```python
from build123d import *

# Parameters (mm, degrees)
ESBO_O1_W                  = 100
ESBO_O1_H                  = 100
RESSALTO_EXTRUS_O1_DEPTH   = 1.5
ESBO_O2_R                  = 1.5
ESBO_O2_W                  = 40
ESBO_O2_H                  = 3
CORTE_EXTRUS_O1_DEPTH      = 71.774289117
ESBO_O3_W                  = 3
ESBO_O3_H                  = 34.5
RESSALTO_EXTRUS_O2_DEPTH   = 3
CUT_EXTRUDE4_DEPTH         = 73.878323252
CUT_EXTRUDE4_DEPTH_BACK    = 73.878323252
FILLET1_R                  = 5
CUT_EXTRUDE5_DEPTH         = 73.878323252
CUT_EXTRUDE5_DEPTH_BACK    = 73.878323252
SKETCH3_W                  = 3
SKETCH3_H                  = 15
SKETCH3_W_2                = 4
SKETCH3_H_2                = 3
SKETCH3_H_3                = 7
CORTE_GY_VL53L0_DEPTH      = 73.924618614
CORTE_GY_VL53L0_DEPTH_BACK = 73.924618614
CUT_EXTRUDE6_DEPTH         = 73.924618614
CUT_EXTRUDE6_DEPTH_BACK    = 73.924618614
SKETCH4_R                  = 1.1
SKETCH4_W                  = 22.5
SKETCH4_H                  = 12.2
CUT_EXTRUDE7_DEPTH         = 73.924618614
CUT_EXTRUDE7_DEPTH_BACK    = 73.924618614


with BuildPart() as part:
    # Esboço1 → Ressalto-extrusão1 (new, symmetric)
    with BuildSketch(Plane.XY):
        Rectangle(ESBO_O1_W, ESBO_O1_H)
    extrude(amount=RESSALTO_EXTRUS_O1_DEPTH, both=True)

    # Esboço2 → Corte-extrusão1 (cut, through all)
    with BuildSketch(Plane.XY.offset(1.5)):
        with Locations((-33, 11.5)):
            Circle(ESBO_O2_R)
        with Locations(Location((33, 11.5, 0), (0, 0, 180))):
            Circle(ESBO_O2_R)
        with Locations((0, -48.5)):
            Rectangle(ESBO_O2_W, ESBO_O2_H)
        with Locations((0, 11.5)):
            Rectangle(ESBO_O2_W, ESBO_O2_H)
    extrude(amount=-CORTE_EXTRUS_O1_DEPTH, mode=Mode.SUBTRACT)

    # Esboço3 → Ressalto-extrusão2 (add, through all)
    with BuildSketch(Plane.XY.offset(1.5)):
        with Locations((-51.5, -32.75)):
            Rectangle(ESBO_O3_W, ESBO_O3_H)
        with Locations((51.5, -32.75)):
            Rectangle(ESBO_O3_W, ESBO_O3_H)
        with Locations((-51.5, 32.75)):
            Rectangle(ESBO_O3_W, ESBO_O3_H)
        with Locations((51.5, 32.75)):
            Rectangle(ESBO_O3_W, ESBO_O3_H)
    extrude(amount=-RESSALTO_EXTRUS_O2_DEPTH)

    # Sketch2 → Cut-Extrude4 (cut, two sides: drawn at the far end of the back side and taken through both)
    with BuildSketch(Plane.XY.offset(-CUT_EXTRUDE4_DEPTH_BACK)):
        with BuildLine():
            Line((-0.5, -35), (0.5, -35))
            ThreePointArc((0.5, -35), (1.207106781, -35.292893219), (1.5, -36))
            Line((1.5, -36), (1.5, -40.73))
            Line((1.5, -40.73), (2.85, -40.73))
            Line((2.85, -40.73), (2.85, -43))
            Line((2.85, -43), (1.5, -43))
            Line((1.5, -43), (1.5, -47))
            Line((1.5, -47), (-1.5, -47))
            Line((-1.5, -47), (-1.5, -43))
            Line((-1.5, -43), (-2.85, -43))
            Line((-2.85, -43), (-2.85, -40.73))
            Line((-2.85, -40.73), (-1.5, -40.73))
            Line((-1.5, -40.73), (-1.5, -36))
            ThreePointArc((-1.5, -36), (-1.207106781, -35.292893219), (-0.5, -35))
        make_face()
    extrude(amount=CUT_EXTRUDE4_DEPTH + CUT_EXTRUDE4_DEPTH_BACK, mode=Mode.SUBTRACT)

    # Fillet1
    fillet1_edges = [part.edges().sort_by_distance(p)[0] for p in [
        (53, 50, 0),
        (-53, 50, 0),
    ]]
    fillet(fillet1_edges, radius=FILLET1_R)

    # Sketch3 → Cut-Extrude5 (cut, two sides: drawn at the far end of the back side and taken through both)
    with BuildSketch(Plane.XY.offset(-CUT_EXTRUDE5_DEPTH_BACK)):
        with Locations((9, -6.5)):
            Rectangle(SKETCH3_W, SKETCH3_H)
        with Locations((9, 28.5)):
            Rectangle(SKETCH3_W, SKETCH3_H)
        with Locations((-9, 28.5)):
            Rectangle(SKETCH3_W, SKETCH3_H)
        with Locations((-9, -6.5)):
            Rectangle(SKETCH3_W, SKETCH3_H)
        with Locations((0, -27.5)):
            Rectangle(SKETCH3_W_2, SKETCH3_H_2)
        Polygon((-15.196152423, -40), (-10, -37), (-8.5, -39.598076211), (-13.696152423, -42.598076211), align=None)
        Polygon((10, -37), (8.5, -39.598076211), (13.696152423, -42.598076211), (15.196152423, -40), align=None)
        with Locations((-48.5, -43.5)):
            Rectangle(SKETCH3_W, SKETCH3_H_3)
        with Locations((48.5, -43.5)):
            Rectangle(SKETCH3_W, SKETCH3_H_3)
    extrude(amount=CUT_EXTRUDE5_DEPTH + CUT_EXTRUDE5_DEPTH_BACK, mode=Mode.SUBTRACT)

    # Sketch1 → Corte Gy-VL53L0 (cut, two sides: drawn at the far end of the back side and taken through both)
    with BuildSketch(Plane(origin=(0, 0, -1.5), x_dir=(-1, 0, 0), z_dir=(0, 0, -1)).offset(-CORTE_GY_VL53L0_DEPTH_BACK)):
        with BuildLine():
            Line((-46.5, 42.530680232), (-46.495662433, 42.530680232))
            ThreePointArc((-46.495662433, 42.530680232), (-46.062649731, 42.780680232), (-46.062649731, 43.280680232))
            Line((-46.062649731, 43.280680232), (-46.64, 44.280680232))
            Line((-46.64, 44.280680232), (-45.07, 47))
            Line((-45.07, 47), (-41.93, 47))
            Line((-41.93, 47), (-40.36, 44.280680232))
            Line((-40.36, 44.280680232), (-40.937350269, 43.280680232))
            ThreePointArc((-40.937350269, 43.280680232), (-40.937350269, 42.780680232), (-40.504337567, 42.530680232))
            Line((-40.504337567, 42.530680232), (-39, 42.530680232))
            ThreePointArc((-39, 42.530680232), (-37.585786438, 41.944893794), (-37, 40.530680232))
            Line((-37, 40.530680232), (-37, 28.530680232))
            ThreePointArc((-37, 28.530680232), (-37.585786438, 27.11646667), (-39, 26.530680232))
            Line((-39, 26.530680232), (-40.504337567, 26.530680232))
            ThreePointArc((-40.504337567, 26.530680232), (-40.937350269, 26.280680232), (-40.937350269, 25.780680232))
            Line((-40.937350269, 25.780680232), (-40.36, 24.780680232))
            Line((-40.36, 24.780680232), (-41.93, 22.061360464))
            Line((-41.93, 22.061360464), (-45.07, 22.061360464))
            Line((-45.07, 22.061360464), (-46.64, 24.780680232))
            Line((-46.64, 24.780680232), (-46.062649731, 25.780680232))
            ThreePointArc((-46.062649731, 25.780680232), (-46.062649731, 26.280680232), (-46.495662433, 26.530680232))
            Line((-46.495662433, 26.530680232), (-48, 26.530680232))
            ThreePointArc((-48, 26.530680232), (-49.414213562, 27.11646667), (-50, 28.530680232))
            Line((-50, 28.530680232), (-50, 34.530680232))
            Line((-50, 34.530680232), (-50, 40.530680232))
            ThreePointArc((-50, 40.530680232), (-49.414213562, 41.944893794), (-48, 42.530680232))
            Line((-48, 42.530680232), (-46.5, 42.530680232))
        make_face()
        with BuildLine():
            Line((46.5, 42.530680232), (46.495662433, 42.530680232))
            ThreePointArc((46.495662433, 42.530680232), (46.062649731, 42.780680232), (46.062649731, 43.280680232))
            Line((46.062649731, 43.280680232), (46.64, 44.280680232))
            Line((46.64, 44.280680232), (45.07, 47))
            Line((45.07, 47), (41.93, 47))
            Line((41.93, 47), (40.36, 44.280680232))
            Line((40.36, 44.280680232), (40.937350269, 43.280680232))
            ThreePointArc((40.937350269, 43.280680232), (40.937350269, 42.780680232), (40.504337567, 42.530680232))
            Line((40.504337567, 42.530680232), (39, 42.530680232))
            ThreePointArc((39, 42.530680232), (37.585786438, 41.944893794), (37, 40.530680232))
            Line((37, 40.530680232), (37, 28.530680232))
            ThreePointArc((37, 28.530680232), (37.585786438, 27.11646667), (39, 26.530680232))
            Line((39, 26.530680232), (40.504337567, 26.530680232))
            ThreePointArc((40.504337567, 26.530680232), (40.937350269, 26.280680232), (40.937350269, 25.780680232))
            Line((40.937350269, 25.780680232), (40.36, 24.780680232))
            Line((40.36, 24.780680232), (41.93, 22.061360464))
            Line((41.93, 22.061360464), (45.07, 22.061360464))
            Line((45.07, 22.061360464), (46.64, 24.780680232))
            Line((46.64, 24.780680232), (46.062649731, 25.780680232))
            ThreePointArc((46.062649731, 25.780680232), (46.062649731, 26.280680232), (46.495662433, 26.530680232))
            Line((46.495662433, 26.530680232), (48, 26.530680232))
            ThreePointArc((48, 26.530680232), (49.414213562, 27.11646667), (50, 28.530680232))
            Line((50, 28.530680232), (50, 34.530680232))
            Line((50, 34.530680232), (50, 40.530680232))
            ThreePointArc((50, 40.530680232), (49.414213562, 41.944893794), (48, 42.530680232))
            Line((48, 42.530680232), (46.5, 42.530680232))
        make_face()
    extrude(amount=CORTE_GY_VL53L0_DEPTH + CORTE_GY_VL53L0_DEPTH_BACK, mode=Mode.SUBTRACT)

    # Sketch4 → Cut-Extrude6 (cut, two sides: drawn at the far end of the back side and taken through both)
    with BuildSketch(Plane.XY.offset(1.5).offset(-CUT_EXTRUDE6_DEPTH_BACK)):
        with Locations((44.15, -2.75)):
            Circle(SKETCH4_R)
        with Locations((16.35, -2.75)):
            Circle(SKETCH4_R)
        with Locations((30.25, -2.75)):
            Rectangle(SKETCH4_W, SKETCH4_H)
    extrude(amount=CUT_EXTRUDE6_DEPTH + CUT_EXTRUDE6_DEPTH_BACK, mode=Mode.SUBTRACT)

    # Sketch6 → Cut-Extrude7 (cut, two sides: drawn at the far end of the back side and taken through both)
    with BuildSketch(Plane.XY.offset(1.5).offset(-CUT_EXTRUDE7_DEPTH_BACK)):
        with BuildLine():
            Line((-31.2, -20.5), (-6.2, -20.5))
            ThreePointArc((-6.2, -20.5), (-4.7, -22), (-6.2, -23.5))
            Line((-6.2, -23.5), (-31.2, -23.5))
            ThreePointArc((-31.2, -23.5), (-32.7, -22), (-31.2, -20.5))
        make_face()
        with BuildLine():
            Line((6.2, -17), (31.2, -17))
            ThreePointArc((31.2, -17), (32.7, -18.5), (31.2, -20))
            Line((31.2, -20), (6.2, -20))
            ThreePointArc((6.2, -20), (4.7, -18.5), (6.2, -17))
        make_face()
    extrude(amount=CUT_EXTRUDE7_DEPTH + CUT_EXTRUDE7_DEPTH_BACK, mode=Mode.SUBTRACT)


solid = part.part
```
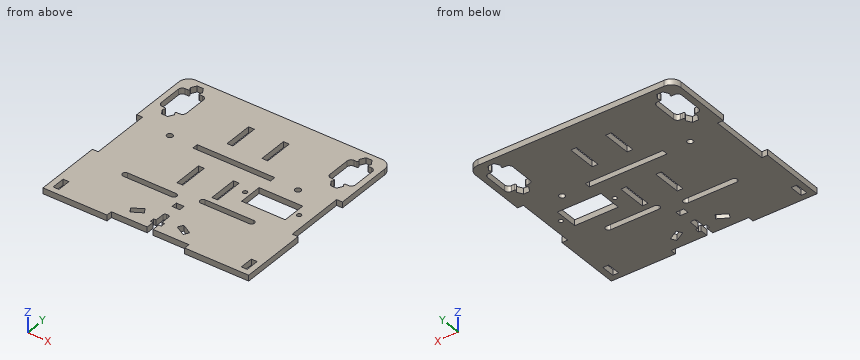
Geometry check sheet. Reference: the model listing, model coordinates, mm. Give positions to 0.01 mm unless a question says otherwise; leave off trailing zeros. Order: outer loops, then holes, each group sorted by start corner. A loop starts at its lowest first (then second) coordinate and runs counter-clockwise, first axis right, second up. Notation, with made-up numbers: (-22.75, -22) - (12.25, -22) arc R25 ccw to (12.25, -7) - close; hole circle Ø2 at (32.5, -9.5). An arc over 180 degrees is marked (long way). Write item = value, one per line. Start each with the question number.
1) Section check C-C (z = 0). Count the separate pieces of the cut face and the enclosed holes in it, then the cut area to 3 significant figures.
2) Section check B-B (y = -27.5). Enter the section's corners in (x, z), then the cut area to 3 significant figures.
3) Section check A-A (y = 11.5). Enter the section's corners in (x, z), then the cut area to 3 significant figures.
4) Scan lines: L1, parallel to Y at x = 44.15, z = -0.15; L2, parallel to X at y = -2.75, z = 0.5; L3, parallel to Y at x = 23.5, z = -0.35. Record each from-to range of solid material in increasing order.
5) Gauge pin test, flat ends, axial feed: pin 1 Ø0.9 at (x, z) = (16.5, 0) entering from -Y; pin 2 Ø0.8 at (x, z) = (0, 0) entering from -Y. Record the tip position at first contact, or that the pin passes through.
Geometry check:
q1.separate_pieces = 1
q1.enclosed_holes = 19
q1.area = 8,890 mm2
q2.outline = (-53, -1.5) - (-2, -1.5) - (-2, 1.5) - (-53, 1.5) - close; (2, -1.5) - (53, -1.5) - (53, 1.5) - (2, 1.5) - close
q2.area = 306 mm2
q3.outline = (-50, -1.5) - (-34.5, -1.5) - (-34.5, 1.5) - (-50, 1.5) - close; (-31.5, -1.5) - (-20, -1.5) - (-20, 1.5) - (-31.5, 1.5) - close; (20, -1.5) - (31.5, -1.5) - (31.5, 1.5) - (20, 1.5) - close; (34.5, -1.5) - (50, -1.5) - (50, 1.5) - (34.5, 1.5) - close
q3.area = 162 mm2
q4.L1 = -50 to -3.85, -1.65 to 22.06, 47 to 50
q4.L2 = -50 to -10.5, -7.5 to 7.5, 10.5 to 15.25, 17.45 to 19, 41.5 to 43.05, 45.25 to 50
q4.L3 = -50 to -20, -17 to -8.85, 3.35 to 50
q5.pin_1 = -47
q5.pin_2 = -35
